```python
from build123d import *

# Parameters (mm, degrees)
BOSS_EXTRUDE1_DEPTH  = 2
BOSS_EXTRUDE6_DEPTH  = 2.5
CUT_EXTRUDE6_DEPTH   = 2.5
BOSS_EXTRUDE14_DEPTH = 2.3
SKETCH32_R           = 2.1
CUT_EXTRUDE7_DEPTH   = 2.3
SKETCH33_W           = 12.5
SKETCH33_H           = 1.343145751
BOSS_EXTRUDE15_DEPTH = 1.2
SKETCH35_W           = 5.479645997
SKETCH35_H           = 5.327993755
CUT_EXTRUDE8_DEPTH   = 2.4
SKETCH36_W           = 3.7
SKETCH36_H           = 1.827993755
CUT_EXTRUDE9_DEPTH   = 2.4
SKETCH37_R           = 3.9
BOSS_EXTRUDE16_DEPTH = 2.3
CUT_EXTRUDE10_DEPTH  = 5.3
SKETCH43_R           = 2.5
BOSS_EXTRUDE17_DEPTH = 1.2
SKETCH44_R           = 0.95
CUT_EXTRUDE11_DEPTH  = 9
SKETCH45_R           = 2
CUT_EXTRUDE12_DEPTH  = 2.5
SKETCH52_R           = 0.75
CUT_EXTRUDE13_DEPTH  = 10


with BuildPart() as part:
    # Sketch3 → Boss-Extrude1 (new body)
    with BuildSketch(Plane.XY):
        with BuildLine():
            Line((8, 0), (9, -2.5))
            Line((9, -2.5), (9, -7))
            Line((9, -7), (21.5, -7))
            Line((21.5, -7), (25.050252532, -4.949747468))
            ThreePointArc((25.050252532, -4.949747468), (36.467156728, -2.678784027), (30, 7))
            Line((30, 7), (27, 7.5))
            Line((27, 7.5), (5.656854249, 7.5))
            Line((5.656854249, 7.5), (5.656854249, 5.656854249))
            ThreePointArc((5.656854249, 5.656854249), (7.39103626, 3.061467459), (8, 0))
        make_face()
    extrude(amount=BOSS_EXTRUDE1_DEPTH)

    # Sketch22 → Boss-Extrude6 (add)
    with BuildSketch(Plane.XY.offset(2)):
        with BuildLine():
            Line((5.656854249, 5.656854249), (2.486790148, 5.656854249))
            Line((2.486790148, 5.656854249), (2.486790148, 7.5))
            Line((2.486790148, 7.5), (5.656854249, 7.5))
            Line((5.656854249, 7.5), (21.5, 7.5))
            Line((21.5, 7.5), (27, 7.5))
            Line((27, 7.5), (27, 2.172006245))
            Line((27, 2.172006245), (23.275126266, 2.172006245))
            Line((23.275126266, 2.172006245), (23.275126266, -5.974873734))
            Line((23.275126266, -5.974873734), (21.5, -7))
            Line((21.5, -7), (9, -7))
            Line((9, -7), (9, -2.5))
            Line((9, -2.5), (8, 0))
            ThreePointArc((8, 0), (7.39103626, 3.061467459), (5.656854249, 5.656854249))
        make_face()
    extrude(amount=BOSS_EXTRUDE6_DEPTH)

    # Sketch26 → Cut-Extrude6 (cut)
    with BuildSketch(Plane.XY.offset(2)):
        Polygon((18.098080448, 5.3), (2.530052458, 5.3), (2.530052458, 4), (18.098080448, 4), (27, 4), (27, 5.3), align=None)
    extrude(amount=CUT_EXTRUDE6_DEPTH, mode=Mode.SUBTRACT)


with BuildPart() as body_2:
    # Sketch31 → Boss-Extrude14 (new body)
    with BuildSketch(Plane.XY.offset(4.5)):
        with BuildLine():
            Line((2.432688066, 5.656854249), (0, 5.656854249))
            ThreePointArc((0, 5.656854249), (-5.656854249, 0), (0, -5.656854249))
            Line((0, -5.656854249), (9, -5.656854249))
            Line((9, -5.656854249), (9, -7))
            Line((9, -7), (21.5, -7))
            Line((21.5, -7), (23.275126266, -5.974873734))
            Line((23.275126266, -5.974873734), (23.275126266, 2.172006245))
            Line((23.275126266, 2.172006245), (27, 2.172006245))
            Line((27, 2.172006245), (27, 7.5))
            Line((27, 7.5), (2.486790148, 7.5))
            Line((2.486790148, 7.5), (2.432688066, 5.656854249))
        make_face()
    extrude(amount=BOSS_EXTRUDE14_DEPTH)

    # Sketch32 → Cut-Extrude7 (cut)
    with BuildSketch(Plane.XY.offset(6.8)):
        Circle(SKETCH32_R)
    extrude(amount=-CUT_EXTRUDE7_DEPTH, mode=Mode.SUBTRACT)

    # Sketch33 → Boss-Extrude15 (add)
    with BuildSketch(Plane.XY.offset(6.8)):
        with Locations((15.25, -6.328427125)):
            Rectangle(SKETCH33_W, SKETCH33_H)
        Polygon((2.486790148, 7.5), (21.5, 7.5), (21.5, 5.656854249), (2.432688066, 5.656854249), align=None)
    extrude(amount=BOSS_EXTRUDE15_DEPTH)


with BuildPart() as cut_extrude8_tool:
    # Sketch35 → Cut-Extrude8 (new body)
    with BuildSketch(Plane.XY.offset(6.8)):
        with Locations((24.260177002, 4.836003123)):
            Rectangle(SKETCH35_W, SKETCH35_H)
    extrude(amount=-CUT_EXTRUDE8_DEPTH)


with BuildPart() as part_1:
    add(part.part)

    # Cut-Extrude8: cut by cut_extrude8_tool
    add(cut_extrude8_tool.part, mode=Mode.SUBTRACT)

    # Sketch36 → Cut-Extrude9 (cut)
    with BuildSketch(Plane.XY.offset(4.4)):
        with Locations((25.15, 3.086003123)):
            Rectangle(SKETCH36_W, SKETCH36_H)
    extrude(amount=-CUT_EXTRUDE9_DEPTH, mode=Mode.SUBTRACT)

    # Sketch37 → Boss-Extrude16 (add)
    with BuildSketch(Plane.XY.offset(2)):
        with Locations((30, 0)):
            Circle(SKETCH37_R)
    extrude(amount=BOSS_EXTRUDE16_DEPTH)

    # Sketch39 → Cut-Extrude10 (cut, through all)
    with BuildSketch(Plane.XY.offset(4.3)):
        with BuildLine():
            Line((29, 1.732050808), (29, -1.732050808))
            ThreePointArc((29, -1.732050808), (32, 0), (29, 1.732050808))
        make_face()
    extrude(amount=-CUT_EXTRUDE10_DEPTH, mode=Mode.SUBTRACT)


with BuildPart() as body_2_1:
    add(body_2.part)

    # Cut-Extrude8: cut by cut_extrude8_tool
    add(cut_extrude8_tool.part, mode=Mode.SUBTRACT)

    # Sketch43 → Boss-Extrude17 (add)
    with BuildSketch(Plane.XY.offset(6.8)):
        with Locations((11.5, 0)):
            Circle(SKETCH43_R)
        with Locations((18, 0)):
            Circle(SKETCH43_R)
    extrude(amount=BOSS_EXTRUDE17_DEPTH)


with BuildPart() as cut_extrude11_tool:
    # Sketch44 → Cut-Extrude11 (new body, through all)
    with BuildSketch(Plane.XY.offset(8)):
        with Locations((11.5, 0)):
            Circle(SKETCH44_R)
        with Locations((18, 0)):
            Circle(SKETCH44_R)
    extrude(amount=-CUT_EXTRUDE11_DEPTH)


with BuildPart() as part_2:
    add(part_1.part)

    # Cut-Extrude11: cut by cut_extrude11_tool
    add(cut_extrude11_tool.part, mode=Mode.SUBTRACT)

    # Sketch45 → Cut-Extrude12 (cut)
    with BuildSketch(Plane(origin=(0, 0, 0), x_dir=(-1, 0, 0), z_dir=(0, 0, -1))):
        with Locations((-11.5, 0)):
            Circle(SKETCH45_R)
        with Locations((-18, 0)):
            Circle(SKETCH45_R)
    extrude(amount=-CUT_EXTRUDE12_DEPTH, mode=Mode.SUBTRACT)


with BuildPart() as body_2_2:
    add(body_2_1.part)

    # Cut-Extrude11: cut by cut_extrude11_tool
    add(cut_extrude11_tool.part, mode=Mode.SUBTRACT)

    # Sketch52 → Cut-Extrude13 (cut, along a direction that is not the sketch's normal)
    with BuildSketch(Plane.XZ.offset(-5.656854249)):
        with Locations((18.235476819, 8)):
            Circle(SKETCH52_R)
    extrude(amount=-CUT_EXTRUDE13_DEPTH, dir=(0.640410196, -0.76803306, 0), mode=Mode.SUBTRACT)


solid = body_2_2.part
```
Read the model definition and answer for the solid it produces. Units are mm, in the model's axes. A direction names the side the tool comes from. Round coordinates to 2 decimals unless told otherwise and drop trailing zeros. Loops run counter-clockwise (first coordinate to the right, second up) from the corner with the lowest first, then second, coordinate; pieces in that order, holes last. Notation, with made-up numbers: (43, -1) -> (49, -1) arc R29 cw to (49, 27) -> close; hole circle Ø3 at (76, -0.75). An arc over 180 degrees is marked (long way). One line per item, written item: value.
1) A cutting plane is placed at B-B (x = 11.5). Determine the outline of the cut face in (y, z).
Answer list:
outline: (-7, 4.5) -> (-0.95, 4.5) -> (-0.95, 8) -> (-2.5, 8) -> (-2.5, 6.8) -> (-5.66, 6.8) -> (-5.66, 8) -> (-7, 8) -> close; (0.95, 4.5) -> (7.5, 4.5) -> (7.5, 8) -> (5.66, 8) -> (5.66, 6.8) -> (2.5, 6.8) -> (2.5, 8) -> (0.95, 8) -> close
2) A cutting plane is placed at D-D (x = 3). Determine the outline of the cut face in (y, z).
Answer list:
outline: (-5.66, 4.5) -> (7.5, 4.5) -> (7.5, 8) -> (5.66, 8) -> (5.66, 6.8) -> (-5.66, 6.8) -> close
3) A cutting plane is placed at A-A (y = 0). Determine the outline of the cut face in (x, z), and give its area (3 significant figures).
Answer list:
outline: (-5.66, 4.5) -> (-2.1, 4.5) -> (-2.1, 6.8) -> (-5.66, 6.8) -> close; (2.1, 4.5) -> (10.55, 4.5) -> (10.55, 8) -> (9, 8) -> (9, 6.8) -> (2.1, 6.8) -> close; (12.45, 4.5) -> (17.05, 4.5) -> (17.05, 8) -> (15.5, 8) -> (15.5, 6.8) -> (14, 6.8) -> (14, 8) -> (12.45, 8) -> close; (18.95, 4.5) -> (23.28, 4.5) -> (23.28, 6.8) -> (20.5, 6.8) -> (20.5, 8) -> (18.95, 8) -> close
area: 55.6 mm²
4) The mould has two halves that part along X. Classify faces 6 (the face through (2.003, 0.631, 5.666)), 7 (the face through (22.38, -6.49, 5.63)), 8 (the face through (12, 7.5, 6)): pulls with the +X half, pulls with the -X half, needs draft (parallel to the pull), parting line crosses it, or undercut.
Answer list:
face 6: undercut
face 7: pulls with the +X half
face 8: needs draft
5) A cutting plane is placed at C-C (z = 6.15). Determine the outline of the cut face in (x, y).
Answer list:
outline: (0, -5.66) -> (9, -5.66) -> (9, -7) -> (21.5, -7) -> (23.28, -5.97) -> (23.28, 2.17) -> (21.52, 2.17) -> (21.52, 7.5) -> (2.49, 7.5) -> (2.43, 5.66) -> (0, 5.66) arc R5.66 ccw to start; hole circle Ø4.2 at (0, 0); hole circle Ø1.9 at (11.5, 0); hole circle Ø1.9 at (18, 0)
6) For faces 1 (the face through (12, 5.657, 7)), 2 (the face through (21.52, 5, 6)), 3 (the face through (1, 5.657, 6)), 4 (the face through (21.5, 7, 7)), 5 (the face through (9, 0, 7)), determine the directions among +Z, -Z, +X, -X, +Y, -Y from which every point of the face is accessible in a straight line to the end or side of a thin tool.
Answer list:
face 1: +Z, +X, -X
face 2: +Z, -Z, +X, +Y
face 3: +Z, -Z, -X, +Y
face 4: +Z, +X, +Y, -Y
face 5: +Z
7) Consider L1, parallel to Y at x = 3, z = 6.7; L2, parallel to Y at x = 12.25, z = 6.3; L3, parallel to Y at x = 4.5, z = 7.4. Determine where each line is inside the solid, lowest interval first. Write a range as [from, to].
Answer list:
L1: y = [-5.66, 7.5]
L2: y = [-7, -0.58], [0.58, 7.5]
L3: y = [5.66, 7.5]
8) Flat-ended cylindrical pins translate along their axes: P1, Ø1, axis at y = 6.5, z = 7.5, coming from the +X side; P2, Ø1.5, axis at x = 1.5, y = -1, coming from the +Z side; P3, Ø0.7, axis at y = -6.5, z = 6, coming from the -X side. Find the tip coordinate at first contact, or state that the pin passes through.
Answer list:
P1: stops at x = 21.5
P2: stops at z = 6.8
P3: stops at x = 9
